from build123d import *

# Parameters (mm, degrees)
F0_R     = 21
F0_R_2   = 20
F1_DEPTH = 2
F2_R     = 21
F2_R_2   = 20
F3_DEPTH = 15
F4_R     = 3.3845023637
F5_DEPTH = 25


# Not quite as in the source:
# - a feature names something its author has since deleted; it is built from what else it names


with BuildPart() as f1:
    # F0 (on Front) → F1 (new body)
    with BuildSketch(Plane.XZ):
        Circle(F0_R)
        Circle(F0_R_2, mode=Mode.SUBTRACT)
        Circle(F0_R_2)
    extrude(amount=-F1_DEPTH)

    # F2 (on face) → F3 (join)
    with BuildSketch(Plane.XZ):
        Circle(F2_R)
        Circle(F2_R_2, mode=Mode.SUBTRACT)
    extrude(amount=F3_DEPTH)

    # F4 (on face) → F5 (cut)
    with BuildSketch(Plane(origin=(0, 2, 0), x_dir=(-1, 0, 0), z_dir=(0, 1, 0))):
        Circle(F4_R)
    extrude(amount=-F5_DEPTH, mode=Mode.SUBTRACT)


solid = f1.part
Build history of the part. All positions in model axes, mm. A direction names the side the tool comes from. Give positions to 0.01 mm unless a question says otherwise; leave off trailing zeros. Order: outer loops, then holes, each group sorted by start corner. A loop starts at its lowest first (then second) coordinate and runs counter-clockwise, first axis right, second up. Notation, with made-up numbers: M 26,-37 L 39,-37 A29 ccw 39,-16 Z; hole C 15,76 d10. An arc over 180 degrees is marked long. Use one line per item in the form item = value.
1) Two-plate mould, pull along Z, no slides. Class faces 1 (the face through (19, -15, -8)), 2 (the face through (4, 0, 0)): released by +Z, released by -Z, zero draft, split by the parting line, or undercut.
Calculated:
face_1 = zero draft
face_2 = undercut
2) Saw through at A-A (x = 0). Give the cut face in (y, z), plus the area to 3 significant figures.
Calculated:
outline = M -15,-21 L 2,-21 L 2,-3.38 L 0,-3.38 L 0,-20 L -15,-20 Z; M -15,20 L 0,20 L 0,3.38 L 2,3.38 L 2,21 L -15,21 Z
area = 100 mm2
3) Saw through at B-B (z = 0). Give the cut face in (x, y).
Calculated:
outline = M -21,-15 L -20,-15 L -20,0 L -3.38,0 L -3.38,2 L -21,2 Z; M 3.38,0 L 20,0 L 20,-15 L 21,-15 L 21,2 L 3.38,2 Z
4) Saw through at D-D (y = -8). Give the cut face in (x, z).
Calculated:
outline = C 0,0 d42; hole C 0,0 d40
5) Drop flat-ended pins along their axis: pin 1 (10 mm diameter, centred on x = -14.5, y = -3.5, fed in from +Z); pin 2 (1.5 mm diameter, centred on y = -6.5, z = -10, fed in from -X); pin 3 (1.5 mm diameter, centred on y = -3, z = -16.5, fed in from -X); pin 4 (8 mm diameter, centred on x = 0, z = 0, fed in from +Y). Give the stop position or say it passes through.
Calculated:
pin_1 = 18.73
pin_2 = -18.85
pin_3 = -13.89
pin_4 = 2
6) Tool access for faces 3 (the face through (-4.336, -7.395, -19.524)), 4 (the face through (4, 2, 0)): list every direction of +Z, -Z, +X, -X, +Y, -Y with a clear straight run to the whole face (end or side of a thin tool).
Calculated:
face_3 = -Y
face_4 = +Z, -Z, +X, -X, +Y
7) Probe probe 1 along Z at (x, y) = (0, -7.75); probe 2 along Z at (x, y) = (0, 0.8); probe 3 along Y at (x, z) = (-10, 9.5). List the from-to ranges inside material, lowest first.
Calculated:
probe_1 = -21 to -20, 20 to 21
probe_2 = -21 to -3.38, 3.38 to 21
probe_3 = 0 to 2
8) Saw through at C-C (z = 13). Give the cut face in (x, y).
Calculated:
outline = M -16.49,-15 L -15.2,-15 L -15.2,0 L 15.2,0 L 15.2,-15 L 16.49,-15 L 16.49,2 L -16.49,2 Z
